Geometry check sheet. Reference: the model listing, model coordinates, mm. A direction names the side the tool comes from. Round coordinates to 2 decimals unless told otherwise and drop trailing zeros. Loops run counter-clockwise (first coordinate to the right, second up) from the corner with the lowest first, then second, coordinate; pieces in that order, holes last. Notation, with made-up numbers: (36, 65.25) -> (52, 65.25) arc R26 ccw to (52, 96.25) -> close; hole circle Ø8 at (56.25, 55). An arc over 180 degrees is marked (long way). Use a Markdown table: item, result. Add a question column.
Q1. Set-up check for faces 4 (the face through (-44.205, -29, -13)), 5 (the face through (-18.805, -19, 6)), 6 (the face through (32, -38.1, 6)): record each of +Z, -Z, +X, -X, +Y, -Y from which the full face is reachable in a straight line by a thin tool's end or side.
Q2. Sectioned sample at C-C, the plane x = 37. Enter the section's corners in (y, z), then the cut area to 3 significant figures.
Q3. Sectioned sample at B-B, the plane y = -11.5. Enter the section's corners in (x, z).
Q4. Gauge pin test, flat end, axial feed: P1, Ø7.5, axis at x = -29, z = 6, coming from the -Y side. Record the tip position at first contact, or that the pin passes through.
Q5. Sectioned sample at D-D, the plane x = -4. Enter the section's corners in (y, z), then the cut area to 3 significant figures.
Q6. Material ranges on L1, parallel to X at y = -29.5, z = 11; L2, parallel to Z at x = 10.5, y = -66.5; L3, parallel to Y at x = 22, z = 11, recorded low to high.
Q7. Release check for a two-part mould opening along X. For faces 1 (the face through (44.695, -29, -13)), 2 (the face through (32, -19, 18.203)), 3 (the face through (19.295, -19, 6)) record: released by +X, released by -X, zero draft, split by the parting line, or undercut.
Q8. Sectioned sample at A-A, the plane z = 7. Enter the section's corners in (x, y).
```python
from build123d import *

# Parameters (mm, degrees)
F0_W     = 88.9
F0_H     = 50.8
F1_DEPTH = 76.2
F3_DEPTH = 25.4


with BuildPart() as f1:
    # F0 (on Front) → F1 (new body)
    with BuildSketch(Plane.XZ):
        with Locations((0.244934, -7.196585)):
            Rectangle(F0_W, F0_H)
    extrude(amount=F1_DEPTH)

    # F2 (on face) → F3 (cut)
    with BuildSketch(Plane.XY.offset(18.203415)):
        Polygon((19.294934, 0), (-18.805066, 0), (-18.805066, -38.1), (-44.205066, -38.1), (-44.205066, -76.2), (44.694934, -76.2), (44.694934, -38.1), (19.294934, -38.1), align=None)
    extrude(amount=-F3_DEPTH, mode=Mode.SUBTRACT)


solid = f1.part
```
Values:
| question | item | result |
|---|---|---|
| 1 | face 4 | +Z, -Z, -X, +Y, -Y |
| 1 | face 5 | +Z, +Y, -Y |
| 1 | face 6 | +Z, +X, -X, -Y |
| 2 | outline | (-76.2, -32.6) -> (0, -32.6) -> (0, 18.2) -> (-38.1, 18.2) -> (-38.1, -7.2) -> (-76.2, -7.2) -> close |
| 2 | area | 2,900 mm^2 |
| 3 | outline | (-44.21, -32.6) -> (44.69, -32.6) -> (44.69, 18.2) -> (19.29, 18.2) -> (19.29, -7.2) -> (-18.81, -7.2) -> (-18.81, 18.2) -> (-44.21, 18.2) -> close |
| 4 | P1 | y = -38.1 |
| 5 | outline | (-76.2, -32.6) -> (0, -32.6) -> (0, -7.2) -> (-76.2, -7.2) -> close |
| 5 | area | 1,940 mm^2 |
| 6 | L1 | -44.21 to -18.81, 19.29 to 44.69 |
| 6 | L2 | -32.6 to -7.2 |
| 6 | L3 | -38.1 to 0 |
| 7 | face 1 | released by +X |
| 7 | face 2 | zero draft |
| 7 | face 3 | undercut |
| 8 | outline | (-44.21, -38.1) -> (-18.81, -38.1) -> (-18.81, 0) -> (-44.21, 0) -> close; (19.29, -38.1) -> (44.69, -38.1) -> (44.69, 0) -> (19.29, 0) -> close |
